Read the model definition and answer for the solid it produces. Units are mm, in the model's axes. A direction names the side the tool comes from. Coordinates: 2 decimals unless noted, no trailing zeros. Loops run counter-clockwise (first coordinate to the right, second up) from the corner with the lowest first, then second, coordinate; pieces in that order, holes last. Notation, with made-up numbers: (76.25, -16.75) -> (96.25, -16.75) arc R29 cw to (96.25, 20.25) -> close; hole circle Ø6 at (-10.5, -23.75). An arc over 180 degrees is marked (long way). Answer in a Markdown table with one row per item.
```python
from build123d import *
from OCP.BRepFilletAPI import BRepFilletAPI_MakeChamfer

# Parameters (mm, degrees)
SKETCH1_W           = 13.97
SKETCH1_H           = 19.05
SKETCH1_R           = 2.413
BOSS_EXTRUDE1_DEPTH = 5.08
SKETCH4_W           = 3.81
SKETCH4_H           = 2.54
BOSS_EXTRUDE4_DEPTH = 6.35
SKETCH5_R           = 4.445
CUT_EXTRUDE1_DEPTH  = 2.54
FILLET2_R           = 0.762
FILLET3_R           = 2.032
CHAMFER2_SIZE       = 0.762
CHAMFER2_SIZE2      = 0.439940905
CHAMFER3_SIZE       = 0.762
CHAMFER3_SIZE2      = 0.439940905
FILLET4_R           = 0.508


with BuildPart() as part:
    # Sketch1 → Boss-Extrude1 (new body)
    with BuildSketch(Plane(origin=(0, 0, 0), x_dir=(1, 0, 0), z_dir=(0, 1, 0))):
        Rectangle(SKETCH1_W, SKETCH1_H)
        with Locations(Location((0, 3.175, 0), (0, 0, 270))):
            Circle(SKETCH1_R, mode=Mode.SUBTRACT)
    extrude(amount=BOSS_EXTRUDE1_DEPTH)

    # Sketch4 → Boss-Extrude4 (add)
    with BuildSketch(Plane.XY.offset(9.525)):
        Polygon((-6.985, 10.16), (-6.985, 7.62), (-3.175, 7.62), (3.175, 7.62), (6.985, 7.62), (6.985, 10.16), align=None)
        with Locations((-5.08, 6.35)):
            Rectangle(SKETCH4_W, SKETCH4_H)
        with Locations((5.08, 6.35)):
            Rectangle(SKETCH4_W, SKETCH4_H)
    extrude(amount=-BOSS_EXTRUDE4_DEPTH)

    # Sketch5 → Cut-Extrude1 (cut)
    with BuildSketch(Plane(origin=(0, 5.08, 0), x_dir=(1, 0, 0), z_dir=(0, 1, 0))):
        with Locations(Location((0, 3.175, 0), (0, 0, 270))):
            Circle(SKETCH5_R)
    extrude(amount=-CUT_EXTRUDE1_DEPTH, mode=Mode.SUBTRACT)

    # Fillet2
    fillet2_edges = [part.edges().sort_by_distance(p)[0] for p in [
        (-6.985, 5.08, -3.175),
        (6.985, 5.08, -3.175),
        (0, 10.16, 3.175),
        (-6.985, 10.16, 6.35),
        (6.985, 7.62, 3.175),
        (6.985, 10.16, 6.35),
        (3.175, 5.08, 6.35),
        (0, 7.62, 3.175),
        (3.175, 7.62, 6.35),
        (-3.175, 6.35, 3.175),
        (-3.175, 7.62, 6.35),
        (-3.175, 5.08, 6.35),
        (-6.985, 7.62, 3.175),
        (5.08, 5.08, 3.175),
        (3.175, 6.35, 3.175),
        (-5.08, 5.08, 3.175),
        (0, 5.08, -7.62),
        (-6.985, 0, 0),
        (0, 0, -9.525),
        (6.985, 0, 0),
        (0, 5.08, -9.525),
    ]]
    fillet(fillet2_edges, radius=FILLET2_R)

    # Fillet3
    # the kernel refuses this fillet: 2.032 mm, written as the material it takes off along each edge
    with BuildSketch(Plane(origin=(-4.953, 5.08, -7.493), x_dir=(0, 0, -1), z_dir=(1, 0, 0))) as fillet3_piece_1:
        with BuildLine():
            CenterArc((1.27, -0.762), 0.762, 0, 90)
            Line((2.032, -0.762), (2.032, 0))
            Line((2.032, 0), (1.27, 0))
        make_face()
    revolve(axis=Axis((-4.953, 5.08, -7.493), (0, 1, 0)), revolution_arc=90, mode=Mode.SUBTRACT)
    with BuildSketch(Plane(origin=(4.953, 5.08, -7.493), x_dir=(1, 0, 0), z_dir=(0, 0, 1))) as fillet3_piece_2:
        with BuildLine():
            CenterArc((1.27, -0.762), 0.762, 0, 90)
            Line((2.032, -0.762), (2.032, 0))
            Line((2.032, 0), (1.27, 0))
        make_face()
    revolve(axis=Axis((4.953, 5.08, -7.493), (0, 1, 0)), revolution_arc=90, mode=Mode.SUBTRACT)
    with BuildSketch(Plane(origin=(-4.953, 0, -7.493), x_dir=(-1, 0, 0), z_dir=(0, 0, 1))) as fillet3_piece_3:
        with BuildLine():
            CenterArc((1.27, -0.762), 0.762, 0, 90)
            Line((2.032, -0.762), (2.032, 0))
            Line((2.032, 0), (1.27, 0))
        make_face()
    revolve(axis=Axis((-4.953, 0, -7.493), (0, -1, 0)), revolution_arc=90, mode=Mode.SUBTRACT)
    with BuildSketch(Plane(origin=(4.953, 0, -7.493), x_dir=(0, 0, -1), z_dir=(-1, 0, 0))) as fillet3_piece_4:
        with BuildLine():
            CenterArc((1.27, -0.762), 0.762, 0, 90)
            Line((2.032, -0.762), (2.032, 0))
            Line((2.032, 0), (1.27, 0))
        make_face()
    revolve(axis=Axis((4.953, 0, -7.493), (0, -1, 0)), revolution_arc=90, mode=Mode.SUBTRACT)
    with BuildSketch(Plane(origin=(6.985, 0, -9.525), x_dir=(0, 0, 1), z_dir=(0, 1, 0))) as fillet3_piece_5:
        with BuildLine():
            CenterArc((FILLET3_R, -FILLET3_R), FILLET3_R, 90, 90)
            Line((0, -FILLET3_R), (0, 0))
            Line((0, 0), (FILLET3_R, 0))
        make_face()
    extrude(amount=5.08, mode=Mode.SUBTRACT)
    with BuildSketch(Plane(origin=(-6.985, 0, -9.525), x_dir=(0, 0, 1), z_dir=(0, 1, 0))) as fillet3_piece_6:
        with BuildLine():
            CenterArc((FILLET3_R, FILLET3_R), FILLET3_R, 180, 90)
            Line((0, FILLET3_R), (0, 0))
            Line((0, 0), (FILLET3_R, 0))
        make_face()
    extrude(amount=5.08, mode=Mode.SUBTRACT)

    # Chamfer2: one chamfer whose edges measure the first distance from different faces: ONE call of the kernel's chamfer builder (chamfer() names one face for all edges)
    chamfer2_edges_1 = [part.edges().sort_by_distance(p)[0] for p in [
        (0, 5.08, 9.525),
    ]]
    chamfer2_side_1 = [part.faces().sort_by_distance(p)[0] for p in [
        (-2.19178656, 5.08, 6.731),
    ]]
    chamfer2_edges_2 = [part.edges().sort_by_distance(p)[0] for p in [
        (3.175, 6.35, 9.525),
    ]]
    chamfer2_side_2 = [part.faces().sort_by_distance(p)[0] for p in [
        (3.175, 6.35, 6.731),
    ]]
    chamfer2_edges_3 = [part.edges().sort_by_distance(p)[0] for p in [
        (-3.175, 6.35, 9.525),
    ]]
    chamfer2_side_3 = [part.faces().sort_by_distance(p)[0] for p in [
        (-3.175, 6.35, 6.731),
    ]]
    chamfer2_edges_4 = [part.edges().sort_by_distance(p)[0] for p in [
        (0, 7.62, 9.525),
    ]]
    chamfer2_side_4 = [part.faces().sort_by_distance(p)[0] for p in [
        (0, 7.62, 6.731),
    ]]
    chamfer2_edges_5 = [part.edges().sort_by_distance(p)[0] for p in [
        (2.951815367, 5.303184633, 9.525),
    ]]
    chamfer2_side_5 = [part.faces().sort_by_distance(p)[0] for p in [
        (2.951815367, 5.303184633, 6.731),
    ]]
    chamfer2_edges_6 = [part.edges().sort_by_distance(p)[0] for p in [
        (-2.951815367, 5.303184633, 9.525),
    ]]
    chamfer2_side_6 = [part.faces().sort_by_distance(p)[0] for p in [
        (-2.951815367, 5.303184633, 6.731),
    ]]
    chamfer2_edges_7 = [part.edges().sort_by_distance(p)[0] for p in [
        (2.951815367, 7.396815367, 9.525),
    ]]
    chamfer2_side_7 = [part.faces().sort_by_distance(p)[0] for p in [
        (2.951815367, 7.396815367, 6.731),
    ]]
    chamfer2_edges_8 = [part.edges().sort_by_distance(p)[0] for p in [
        (-2.951815367, 7.396815367, 9.525),
    ]]
    chamfer2_side_8 = [part.faces().sort_by_distance(p)[0] for p in [
        (-2.951815367, 7.396815367, 6.731),
    ]]
    chamfer2 = BRepFilletAPI_MakeChamfer(part.part.solid().wrapped)
    for e in chamfer2_edges_1:
        chamfer2.Add(CHAMFER2_SIZE, CHAMFER2_SIZE2, e.wrapped, chamfer2_side_1[0].wrapped)  # the first distance lies on this face
    for e in chamfer2_edges_2:
        chamfer2.Add(CHAMFER2_SIZE, CHAMFER2_SIZE2, e.wrapped, chamfer2_side_2[0].wrapped)  # the first distance lies on this face
    for e in chamfer2_edges_3:
        chamfer2.Add(CHAMFER2_SIZE, CHAMFER2_SIZE2, e.wrapped, chamfer2_side_3[0].wrapped)  # the first distance lies on this face
    for e in chamfer2_edges_4:
        chamfer2.Add(CHAMFER2_SIZE, CHAMFER2_SIZE2, e.wrapped, chamfer2_side_4[0].wrapped)  # the first distance lies on this face
    for e in chamfer2_edges_5:
        chamfer2.Add(CHAMFER2_SIZE, CHAMFER2_SIZE2, e.wrapped, chamfer2_side_5[0].wrapped)  # the first distance lies on this face
    for e in chamfer2_edges_6:
        chamfer2.Add(CHAMFER2_SIZE, CHAMFER2_SIZE2, e.wrapped, chamfer2_side_6[0].wrapped)  # the first distance lies on this face
    for e in chamfer2_edges_7:
        chamfer2.Add(CHAMFER2_SIZE, CHAMFER2_SIZE2, e.wrapped, chamfer2_side_7[0].wrapped)  # the first distance lies on this face
    for e in chamfer2_edges_8:
        chamfer2.Add(CHAMFER2_SIZE, CHAMFER2_SIZE2, e.wrapped, chamfer2_side_8[0].wrapped)  # the first distance lies on this face
    add(Compound.cast(chamfer2.Shape()), mode=Mode.REPLACE)

    # Chamfer3: one chamfer whose edges measure the first distance from different faces: ONE call of the kernel's chamfer builder (chamfer() names one face for all edges)
    chamfer3_edges_1 = [part.edges().sort_by_distance(p)[0] for p in [
        (6.985, 5.08, 9.525),
    ]]
    chamfer3_side_1 = [part.faces().sort_by_distance(p)[0] for p in [
        (6.985, 3.922875555, 2.845032122),
    ]]
    chamfer3_edges_2 = [part.edges().sort_by_distance(p)[0] for p in [
        (-6.985, 5.08, 9.525),
    ]]
    chamfer3_side_2 = [part.faces().sort_by_distance(p)[0] for p in [
        (-6.985, 3.922875555, 2.845032122),
    ]]
    chamfer3_edges_3 = [part.edges().sort_by_distance(p)[0] for p in [
        (0, 0, 9.525),
    ]]
    chamfer3_side_3 = [part.faces().sort_by_distance(p)[0] for p in [
        (0, 0, 0.722183851),
    ]]
    chamfer3_edges_4 = [part.edges().sort_by_distance(p)[0] for p in [
        (0, 10.16, 9.525),
    ]]
    chamfer3_side_4 = [part.faces().sort_by_distance(p)[0] for p in [
        (0, 10.16, 6.731),
    ]]
    chamfer3_edges_5 = [part.edges().sort_by_distance(p)[0] for p in [
        (6.761815367, 9.936815367, 9.525),
    ]]
    chamfer3_side_5 = [part.faces().sort_by_distance(p)[0] for p in [
        (6.761815367, 9.936815367, 6.731),
    ]]
    chamfer3_edges_6 = [part.edges().sort_by_distance(p)[0] for p in [
        (-6.761815367, 9.936815367, 9.525),
    ]]
    chamfer3_side_6 = [part.faces().sort_by_distance(p)[0] for p in [
        (-6.761815367, 9.936815367, 6.731),
    ]]
    chamfer3_edges_7 = [part.edges().sort_by_distance(p)[0] for p in [
        (-6.761815367, 0.223184633, 9.525),
    ]]
    chamfer3_side_7 = [part.faces().sort_by_distance(p)[0] for p in [
        (-6.761815367, 0.223184633, 1.016),
    ]]
    chamfer3_edges_8 = [part.edges().sort_by_distance(p)[0] for p in [
        (6.761815367, 0.223184633, 9.525),
    ]]
    chamfer3_side_8 = [part.faces().sort_by_distance(p)[0] for p in [
        (6.761815367, 0.223184633, 1.016),
    ]]
    chamfer3 = BRepFilletAPI_MakeChamfer(part.part.solid().wrapped)
    for e in chamfer3_edges_1:
        chamfer3.Add(CHAMFER3_SIZE, CHAMFER3_SIZE2, e.wrapped, chamfer3_side_1[0].wrapped)  # the first distance lies on this face
    for e in chamfer3_edges_2:
        chamfer3.Add(CHAMFER3_SIZE, CHAMFER3_SIZE2, e.wrapped, chamfer3_side_2[0].wrapped)  # the first distance lies on this face
    for e in chamfer3_edges_3:
        chamfer3.Add(CHAMFER3_SIZE, CHAMFER3_SIZE2, e.wrapped, chamfer3_side_3[0].wrapped)  # the first distance lies on this face
    for e in chamfer3_edges_4:
        chamfer3.Add(CHAMFER3_SIZE, CHAMFER3_SIZE2, e.wrapped, chamfer3_side_4[0].wrapped)  # the first distance lies on this face
    for e in chamfer3_edges_5:
        chamfer3.Add(CHAMFER3_SIZE, CHAMFER3_SIZE2, e.wrapped, chamfer3_side_5[0].wrapped)  # the first distance lies on this face
    for e in chamfer3_edges_6:
        chamfer3.Add(CHAMFER3_SIZE, CHAMFER3_SIZE2, e.wrapped, chamfer3_side_6[0].wrapped)  # the first distance lies on this face
    for e in chamfer3_edges_7:
        chamfer3.Add(CHAMFER3_SIZE, CHAMFER3_SIZE2, e.wrapped, chamfer3_side_7[0].wrapped)  # the first distance lies on this face
    for e in chamfer3_edges_8:
        chamfer3.Add(CHAMFER3_SIZE, CHAMFER3_SIZE2, e.wrapped, chamfer3_side_8[0].wrapped)  # the first distance lies on this face
    add(Compound.cast(chamfer3.Shape()), mode=Mode.REPLACE)

    # Fillet4
    fillet4_edges = [part.edges().sort_by_distance(p)[0] for p in [
        (0, 2.54, -5.588),
    ]]
    fillet(fillet4_edges, radius=FILLET4_R)


solid = part.part
```
1. A cutting plane is placed at C-C on y = 6.5. Give the vertices of the cut face in (x, z) (3 decimals).
A:
| item | result |
|---|---|
| outline | (-6.985, 3.937) arc R0.762 ccw to (-6.223, 3.175) -> (-3.937, 3.175) arc R0.762 ccw to (-3.175, 3.937) -> (-3.175, 8.763) -> (-3.615, 9.525) -> (-6.545, 9.525) -> (-6.985, 8.763) -> close; (3.175, 3.937) arc R0.762 ccw to (3.937, 3.175) -> (6.223, 3.175) arc R0.762 ccw to (6.985, 3.937) -> (6.985, 8.763) -> (6.545, 9.525) -> (3.615, 9.525) -> (3.175, 8.763) -> close |
2. The mould has two halves that part along X. Classify faces 1 (the cylindrical face through (-6.37, 2.52, -8.95)), 2 (the conical face through (-3.102, 7.562, 9.149)), 3 (the flat face through (0, 9, 3.175)): pulls with the +X half, pulls with the -X half, needs draft (parallel to the pull), parting line crosses it, or undercut.
A:
| item | result |
|---|---|
| face 1 | pulls with the -X half |
| face 2 | undercut |
| face 3 | needs draft |
3. A cutting plane is placed at A-A on x = 0. Give the vertices of the cut face in (y, z) (3 decimals).
A:
| item | result |
|---|---|
| outline | (0, -8.763) arc R0.762 ccw to (0.762, -9.525) -> (4.318, -9.525) arc R0.762 ccw to (5.08, -8.763) -> (5.08, -8.382) arc R0.762 ccw to (4.318, -7.62) -> (2.54, -7.62) -> (2.54, -6.096) arc R0.508 ccw to (2.032, -5.588) -> (0, -5.588) -> close; (0, -0.762) -> (2.032, -0.762) arc R0.508 ccw to (2.54, -0.254) -> (2.54, 1.27) -> (4.318, 1.27) arc R0.762 ccw to (5.08, 2.032) -> (5.08, 8.763) -> (4.64, 9.525) -> (0.44, 9.525) -> (0, 8.763) -> close; (7.62, 3.937) arc R0.762 ccw to (8.382, 3.175) -> (9.398, 3.175) arc R0.762 ccw to (10.16, 3.937) -> (10.16, 8.763) -> (9.72, 9.525) -> (8.06, 9.525) -> (7.62, 8.763) -> close |
4. Given pin 1 Ø4.5 at (x, z) = (0, -3.175) entering from -Y; pin 2 Ø8 at (x, z) = (0, -3.175) entering from +Y; pin 3 Ø1.8 at (x, y) = (0, 7) entering from -Z; pin 4 Ø1 at (x, z) = (3, -6.5) entering from +Y, each flat-ended and moving along its own axis, determine where each tip first touches the part or whether it passes through.
A:
| item | result |
|---|---|
| pin 1 | passes through |
| pin 2 | stops at y = 2.54 |
| pin 3 | stops at z = 3.35 |
| pin 4 | stops at y = 5.04 |
5. A tool of negligible diameter and unlimited length cuts with its end or side. For faces 4 (the conical face through (-3.117, 5.153, 9.149)), 5 (the flat face through (0, 7.62, 6)), 6 (the cylindrical face through (-4.34, 3.44, -4.14)), 7 (the flat face through (-3, 5.08, 2)), from which of +Z, -Z, +X, -X, +Y, -Y can it reach the whole face along a straight path? Write none if from no direction.
A:
| item | result |
|---|---|
| face 4 | +Z |
| face 5 | +Z, -Z |
| face 6 | +Y |
| face 7 | -Z |
6. Find the intervals of material crossed by probe 1 along Z at (x, y) = (0, 0.75) (3 decimals); probe 2 along Y at (x, z) = (0, 7.5); probe 3 along Y at (x, z) = (6, -1.5), in increasing order.
A:
| item | result |
|---|---|
| probe 1 | z = -9.525 to -5.588, -0.762 to 9.525 |
| probe 2 | y = 0 to 5.08, 7.62 to 10.16 |
| probe 3 | y = 0 to 5.08 |
7. A cutting plane is placed at B-B on z = 4.25. Give the vertices of the cut face in (x, y) (3 decimals), and give its area (3 significant figures).
A:
| item | result |
|---|---|
| outline | (-6.985, 0.762) arc R0.762 ccw to (-6.223, 0) -> (6.223, 0) arc R0.762 ccw to (6.985, 0.762) -> (6.985, 9.398) arc R0.762 ccw to (6.223, 10.16) -> (-6.223, 10.16) arc R0.762 ccw to (-6.985, 9.398) -> close; hole (-3.175, 5.842) arc R0.762 ccw to (-2.413, 5.08) -> (2.413, 5.08) arc R0.762 ccw to (3.175, 5.842) -> (3.175, 6.858) arc R0.762 ccw to (2.413, 7.62) -> (-2.413, 7.62) arc R0.762 ccw to (-3.175, 6.858) -> close |
| area | 126 mm2 |
